Check sheet for the drawn part. Datum: minimum x, y, z corner. Units: mm. Give positions to 0.01 mm unless a question says otherwise; leave off trailing zeros. Write each loop counter-clockwise with the first axis right and the second up, starting at its lowest first coordinate (ties: lowest second). Pieces come first, ordered by that corner, then holes. Notation, with made-up numbers: (-4, -11) - (0, -11) arc R14 ccw to (0, 13) - close; hole circle Ø7 at (24, 87). An arc over 180 degrees is marked (long way). One line per question, with ' | ' between items. Start each with the question number.
Q1. Release check for a two-part mould opening along X. For the marked faces 1, 2 and 3 record: +X half, -X half, draft (parallel to the pull), parting line (faces both ways), or undercut.
Q2. Section check A-A on x = 34.5. Record the boundary of the cut face in (y, z), and give its area (3 significant figures).
Q3. Gauge pin test, flat ends, axial feed: P1, Ø2, axis at y = 2, z = 48.5, coming from the -X side; P2, Ø1.5, axis at x = 28.5, z = 119.5, coming from the -Y side; P3, Ø1, axis at x = 57.5, z = 101, coming from the +Y side; P4, Ø10, axis at x = 97.5, z = 185.5, coming from the +Y side. Record the tip position at first contact, or that the pin passes through.
Q4. Thickness scan on L1, parallel to X at y = 4.5, z = 109.5; L2, parallel to X at y = 4.75, z = 147; L3, parallel to Z at x = 83, y = 10.25. Record the ranges inside material, lowest first. Write a range as [from, to].
Q5. Section check C-C on z = 100. Record the boundary of the cut face in (x, y), and give its area (3 significant figures).
Q6. Section check B-B on y = 7.5. Record the boundary of the cut face in (x, z) (1 decimal).
Q7. Section check D-D on x = 107. Record the boundary of the cut face in (y, z).
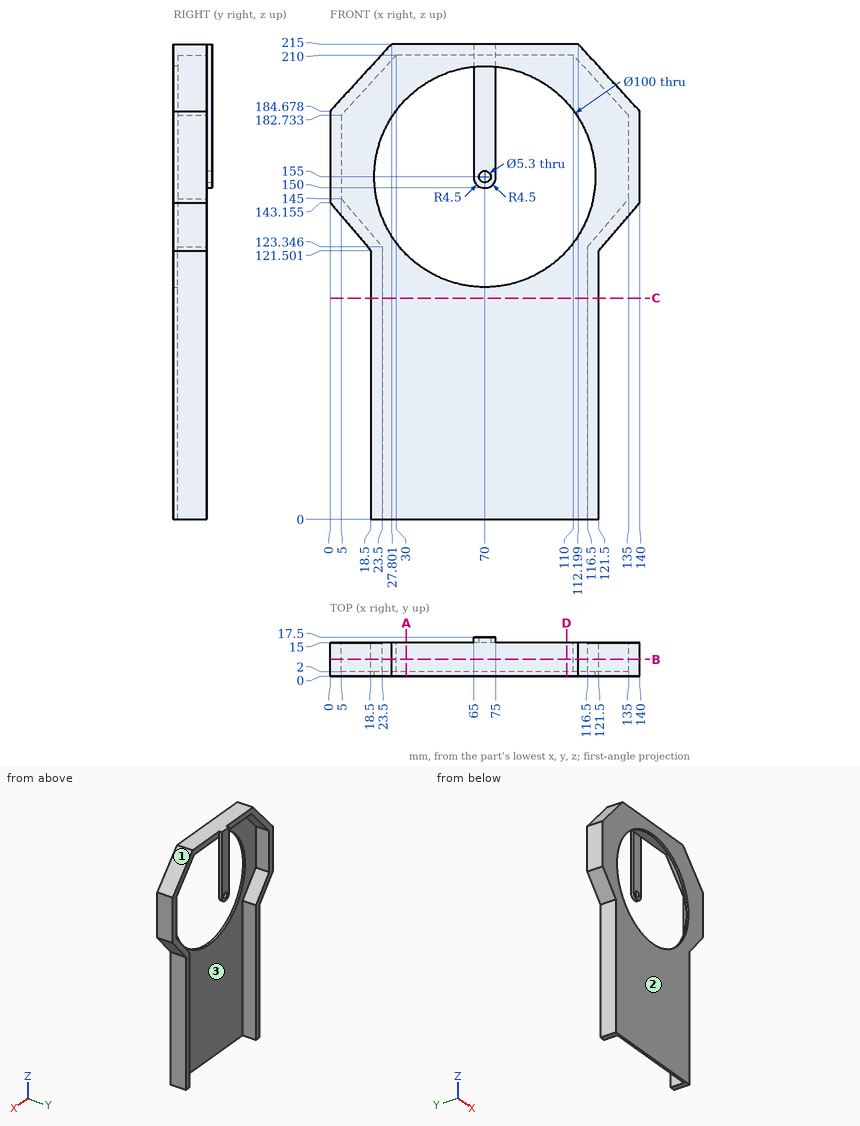
Working result:
1) face 1: +X half | face 2: draft | face 3: undercut
2) outline: (0, 0) - (2, 0) - (2, 119.79) - (0, 119.79) - close; (0, 190.21) - (2, 190.21) - (2, 210) - (15, 210) - (15, 215) - (0, 215) - close | area: 354 mm2
3) P1: stops at x = 18.5 | P2: stops at y = 0 | P3: stops at y = 2 | P4: passes through
4) L1: x = [18.5, 23.5], [116.5, 121.5] | L2: x = [0, 5], [135, 140] | L3: z = [210, 215]
5) outline: (18.5, 0) - (121.5, 0) - (121.5, 15) - (116.5, 15) - (116.5, 2) - (23.5, 2) - (23.5, 15) - (18.5, 15) - close | area: 336 mm2
6) outline: (0, 143.2) - (18.5, 121.5) - (18.5, 0) - (23.5, 0) - (23.5, 123.3) - (5, 145) - (5, 182.7) - (30, 210) - (110, 210) - (135, 182.7) - (135, 145) - (116.5, 123.3) - (116.5, 0) - (121.5, 0) - (121.5, 121.5) - (140, 143.2) - (140, 184.7) - (112.2, 215) - (27.8, 215) - (0, 184.7) - close
7) outline: (0, 0) - (2, 0) - (2, 121.37) - (0, 121.37) - close; (0, 188.63) - (2, 188.63) - (2, 210) - (15, 210) - (15, 215) - (0, 215) - close
